from build123d import *

# Parameters (mm, degrees)
PAD_DEPTH = 1


with BuildPart() as part:
    # Sketch007 → Pad (new body)
    with BuildSketch(Plane.XY):
        with BuildLine():
            ThreePointArc((28.5, 19.015221), (27.202361, 21.964331), (24.151377, 23))
            Line((18.403463, 22.497123), (24.151377, 23))
            ThreePointArc((18.403463, 22.497123), (16.638159, 21.720371), (15.710507, 20.029483))
            Line((15.710507, 20.029483), (15, 16))
            Line((15, 16), (15, 0))
            Line((15, 0), (28, 0))
            Line((28, 0), (28, 10.677124))
            ThreePointArc((28.25, 11.338562), (28.064586, 11.030678), (28, 10.677124))
            ThreePointArc((28.25, 11.338562), (28.435414, 11.646447), (28.5, 12))
            Line((28.5, 19.015221), (28.5, 12))
        make_face()
    pad = extrude(amount=PAD_DEPTH)

    # Mirrored: Pad across Sketch007 H_Axis
    add(pad.mirror(Plane.ZX))


solid = part.part
Input: part model. Units: mm. Frame: model coordinates. Coordinates: 2 decimals unless noted, no trailing zeros. Loops run counter-clockwise (first coordinate to the right, second up) from the corner with the lowest first, then second, coordinate; pieces in that order, holes last. Notation, with made-up numbers: (40.25, 32.25) -> (65.25, 32.25) arc R24 ccw to (65.25, 71.25) -> close; hole circle Ø1 at (-10.75, 25.25). An arc over 180 degrees is marked (long way). One line per item, written item: value.
(1) Cut plane A-A (z = 0.85). Output: boundary loops of the cut face in (x, y), then the cut area to 3 significant figures.
Answer below:
outline: (15, -16) -> (15.71, -20.03) arc R3 ccw to (18.4, -22.5) -> (24.15, -23) arc R4 ccw to (28.5, -19.02) -> (28.5, -12) arc R1 ccw to (28.25, -11.34) arc R1 cw to (28, -10.68) -> (28, 10.68) arc R1 cw to (28.25, 11.34) arc R1 ccw to (28.5, 12) -> (28.5, 19.02) arc R4 ccw to (24.15, 23) -> (18.4, 22.5) arc R3 ccw to (15.71, 20.03) -> (15, 16) -> close
area: 587 mm2
(2) Cut plane B-B (y = 18). Output: boundary loops of the cut face in (x, z).
Answer below:
outline: (15.35, 0) -> (28.5, 0) -> (28.5, 1) -> (15.35, 1) -> close
(3) Cut plane C-C (x = 16.25). Output: boundary loops of the cut face in (y, z).
Answer below:
outline: (-21.29, 0) -> (21.29, 0) -> (21.29, 1) -> (-21.29, 1) -> close
(4) Ray query, line 1 along X through (y, z) = (-10, 0.15); line 2 along Y through (x, z) = (24.25, 0.35); line 3 along Y through (x, z) = (27.75, 0.65). Return the intervals inside material, ascending.
Answer below:
line 1: x = 15 to 28
line 2: y = -23.01 to 23.01
line 3: y = -21.35 to 21.35
(5) Draft query along Y for faces 1 (the face through (28, 0.1, 0.5)), 2 (the face through (15.36, 18.04, 0.49)), 3 (the face through (22, 0, 0)). Return one class per face: pulls with the +Y half, pulls with the -Y half, needs draft (parallel to the pull), parting line crosses it, or undercut.
Answer below:
face 1: undercut
face 2: pulls with the +Y half
face 3: needs draft
